Part model, mm, in its own coordinate system. Coordinates: 2 decimals unless noted, no trailing zeros. Answer as a JSON object with one key per item and string values. Group by question number.
1. Drill centre lines: L1, parallel to X at y = 2.7, z = -40; L2, parallel to X at y = 5.4, z = -21.5; L3, parallel to Z at x = -8.5, y = 5.4. Where is each one in solid material? Low to high.
2. Drop a flat-ended pin along its axis: pin 1 Ø8 at (x, z) = (0, -60) entering from +Y. Give the stop position or say it passes through.
3. Saw through at A-A on y = 2.1. Count the separate pieces of the cut face and the enclosed holes in it, then the cut area to 3 significant figures.
from build123d import *

# Parameters (mm, degrees)
SKETCH_1_R      = 3
EXTRUDE_1_DEPTH = 6


with BuildPart() as part:
    # Эскиз1 → Бобышка-Вытянуть1 (new body)
    with BuildSketch(Plane(origin=(0, 0, 0), x_dir=(1, 0, 0), z_dir=(0, 1, 0))):
        with BuildLine():
            Line((-15, -300), (-3, -300))
            Line((-3, -300), (-3, -285))
            Line((-3, -285), (3, -285))
            Line((3, -285), (3, -300))
            Line((3, -300), (15, -300))
            Line((15, -300), (15, 300))
            ThreePointArc((15, 300), (0, 315), (-15, 300))
            Line((-15, 300), (-15, -300))
        make_face()
        with Locations((0, 300)):
            Circle(SKETCH_1_R, mode=Mode.SUBTRACT)
        with Locations((0, 280)):
            Circle(SKETCH_1_R, mode=Mode.SUBTRACT)
        with Locations((0, 260)):
            Circle(SKETCH_1_R, mode=Mode.SUBTRACT)
        with Locations((0, 240)):
            Circle(SKETCH_1_R, mode=Mode.SUBTRACT)
        with Locations((0, 220)):
            Circle(SKETCH_1_R, mode=Mode.SUBTRACT)
        with Locations((0, 200)):
            Circle(SKETCH_1_R, mode=Mode.SUBTRACT)
        with Locations((0, 180)):
            Circle(SKETCH_1_R, mode=Mode.SUBTRACT)
        with Locations((0, 160)):
            Circle(SKETCH_1_R, mode=Mode.SUBTRACT)
        with Locations((0, 140)):
            Circle(SKETCH_1_R, mode=Mode.SUBTRACT)
        with Locations((0, 120)):
            Circle(SKETCH_1_R, mode=Mode.SUBTRACT)
        with Locations((0, 100)):
            Circle(SKETCH_1_R, mode=Mode.SUBTRACT)
        with Locations((0, 80)):
            Circle(SKETCH_1_R, mode=Mode.SUBTRACT)
        with Locations((0, 60)):
            Circle(SKETCH_1_R, mode=Mode.SUBTRACT)
        with Locations((0, 40)):
            Circle(SKETCH_1_R, mode=Mode.SUBTRACT)
        with Locations((0, 20)):
            Circle(SKETCH_1_R, mode=Mode.SUBTRACT)
        Circle(SKETCH_1_R, mode=Mode.SUBTRACT)
        with Locations((0, -20)):
            Circle(SKETCH_1_R, mode=Mode.SUBTRACT)
        with Locations((0, -40)):
            Circle(SKETCH_1_R, mode=Mode.SUBTRACT)
        with Locations((0, -60)):
            Circle(SKETCH_1_R, mode=Mode.SUBTRACT)
        with Locations((0, -80)):
            Circle(SKETCH_1_R, mode=Mode.SUBTRACT)
        with Locations((0, -100)):
            Circle(SKETCH_1_R, mode=Mode.SUBTRACT)
        with Locations((0, -120)):
            Circle(SKETCH_1_R, mode=Mode.SUBTRACT)
        with Locations((0, -140)):
            Circle(SKETCH_1_R, mode=Mode.SUBTRACT)
        with Locations((0, -160)):
            Circle(SKETCH_1_R, mode=Mode.SUBTRACT)
        with Locations((0, -180)):
            Circle(SKETCH_1_R, mode=Mode.SUBTRACT)
        with Locations((0, -200)):
            Circle(SKETCH_1_R, mode=Mode.SUBTRACT)
        with Locations((0, -220)):
            Circle(SKETCH_1_R, mode=Mode.SUBTRACT)
        with Locations((0, -240)):
            Circle(SKETCH_1_R, mode=Mode.SUBTRACT)
    extrude(amount=EXTRUDE_1_DEPTH)


solid = part.part
Outcome:
{
 "1": {"L1": "x = -15 to -3, 3 to 15", "L2": "x = -15 to -2.6, 2.6 to 15", "L3": "z = -312.36 to 300"},
 "2": {"pin 1": "stops at y = 6"},
 "3": {"separate pieces": "1", "enclosed holes": "28", "area": "17,500 mm²"}
}
